Autodesk Inventor part; units mm, degrees
ref_plane "YZ Plane" through (0, 0, 0) normal (1, 0, 0) x (0, 1, 0)
ref_plane "XZ Plane" through (0, 0, 0) normal (0, 1, 0) x (-1, 0, 0)
ref_plane "XY Plane" through (0, 0, 0) normal (0, 0, 1) x (1, 0, 0)
sketch "Sketch1" plane through (0, 0, 0) normal (0, 0, 1) x (1, 0, 0)
  line L0 (0, 0) -> (3.175, 0)
  line L1 (3.175, 0) -> (3.175, 50.8)
  line L2 (3.175, 50.8) -> (0, 50.8)
  line L3 (0, 50.8) -> (0, 0)
  line L4 (0, 0) -> (50.8, 0)
  line L5 (50.8, 0) -> (50.8, 3.175)
  line L6 (50.8, 3.175) -> (0, 3.175)
  line L7 (0, 3.175) -> (0, 0)
  dimension "d0" = 3.175
  dimension "d1" = 50.8
  dimension "d2" = 50.8
  dimension "d3" = 3.175
extrude "Extrusion1" add sketch "Sketch1" along normal blind 25.4
sketch "Sketch2" plane through (3.175, 3.175, 0) normal (1, 0, 0) x (0, 0, -1)
  line L0 (0, 47.625) -> (-25.4, 47.625) construction
  line L1 (0, 0) -> (-25.4, 0) construction
  line L2 (-12.7, 0) -> (-12.7, 9.525) construction
  circle A0 centre (-12.7, 9.525) radius 2.5797
  line L3 (-12.7, 9.525) -> (-12.7, 34.925) construction
  circle A1 centre (-12.7, 34.925) radius 2.5797
  point P0 (0, -3.175)
  dimension "d18" = 9.525
  dimension "d19" = 5.1594
  dimension "d22" = 25.4
  dimension "d23" = 5.1594
extrude "Extrusion2" cut sketch "Sketch2" against normal blind 25.4
sketch "Sketch3" plane through (3.175, 3.175, 0) normal (0, 1, 0) x (1, 0, 0)
  line L0 (0, 0) -> (0, -25.4) construction
  line L1 (0, -12.7) -> (9.525, -12.7) construction
  circle A0 centre (9.525, -12.7) radius 2.5797
  line L2 (9.525, -12.7) -> (34.925, -12.7) construction
  circle A1 centre (34.925, -12.7) radius 2.5797
  point P0 (-3.175, 0)
  dimension "d12" = 9.525
  dimension "d13" = 5.1594
  dimension "d14" = 25.4
  dimension "d15" = 5.1594
extrude "Extrusion3" cut sketch "Sketch3" against normal blind 25.4
properties part number "LV Gusset"
Here's how the part is built. I have some questions about the finished solid (model axes, mm). A direction names the side the tool comes from. Coordinates: 2 decimals unless noted, no trailing zeros. Order: outer loops, then holes, each group sorted by start corner. A loop starts at its lowest first (then second) coordinate and runs counter-clockwise, first axis right, second up.
Item 1: For faces 1 (the face through (40.561, 1.61, 11.925)), 2 (the face through (3.175, 27, 13)), which set-ups out of +Z, -Z, +X, -X, +Y, -Y let a thin tool reach every point of the face, with its end or its side?
Result sheet:
face 1: +Y, -Y
face 2: +Z, -Z, +X, +Y
Item 2: If we section it at D-D on z = 19: List the corners of the cut face in (x, y) for me (3 decimals), plus the area to 4 significant figures.
Result sheet:
outline: (0, 0) - (50.8, 0) - (50.8, 3.175) - (3.175, 3.175) - (3.175, 50.8) - (0, 50.8) - close
area: 312.5 mm2
Item 3: If we section it at C-C on x = 14: List the corners of the cut face in (y, z) for me (3 decimals).
Result sheet:
outline: (0, 0) - (3.175, 0) - (3.175, 10.472) - (0, 10.472) - close; (0, 14.928) - (3.175, 14.928) - (3.175, 25.4) - (0, 25.4) - close
Item 4: For P1, Ø7.5, axis at y = 26.5, z = 13.5, coming from the +X side (3 decimals); P2, Ø12.5, axis at x = 27.5, z = 8.5, coming from the +Y side (3 decimals), each with a flat end and sliding along its axis, tell me the tip position at first contact or that it passes through.
Result sheet:
P1: stops at x = 3.175
P2: stops at y = 3.175
Item 5: I need wall thicknesses on line 1 (Y direction, x = 1.9, z = 12.7); line 2 (Z direction, x = 12.7, y = 2.3). Which ranges of each line are inside material? Lowest first, please.
Result sheet:
line 1: y = 0 to 10.12, 15.28 to 35.52, 40.68 to 50.8
line 2: z = 0 to 10.12, 15.28 to 25.4
Item 6: If we section it at A-A on z = 12.7: List the corners of the cut face in (x, y) for me (3 decimals).
Result sheet:
outline: (0, 0) - (10.12, 0) - (10.12, 3.175) - (3.175, 3.175) - (3.175, 10.12) - (0, 10.12) - close; (0, 15.28) - (3.175, 15.28) - (3.175, 35.52) - (0, 35.52) - close; (0, 40.68) - (3.175, 40.68) - (3.175, 50.8) - (0, 50.8) - close; (15.28, 0) - (35.52, 0) - (35.52, 3.175) - (15.28, 3.175) - close; (40.68, 0) - (50.8, 0) - (50.8, 3.175) - (40.68, 3.175) - close
Item 7: If we section it at B-B on y = 12.7: List the corners of the cut face in (x, z) for me (3 decimals), plus the area to 3 significant figures.
Result sheet:
outline: (0, 0) - (3.175, 0) - (3.175, 10.12) - (0, 10.12) - close; (0, 15.28) - (3.175, 15.28) - (3.175, 25.4) - (0, 25.4) - close
area: 64.3 mm2
Item 8: If we mould it in two halves opening along Z, with no side actions, what happens to faces 3 (the face through (1.61, 35.81, 11.51)), 4 (the face through (3, 14, 25.4)), 5 (the face through (2, 50.8, 13)), 6 (the face through (3, 14, 0))? For each: +Z half, -Z half, draft (parallel to the pull), parting line (faces both ways), or undercut.
Result sheet:
face 3: undercut
face 4: +Z half
face 5: draft
face 6: -Z half
